Geometry: see drawing. Coordinates: mm, zero at the bounding-box minimum. A direction names the side the tool comes from. Round coordinates to 2 decimals unless told otherwise and drop trailing zeros. Loops run counter-clockwise (first coordinate to the right, second up) from the corner with the lowest first, then second, coordinate; pieces in that order, holes last. Notation, with made-up numbers: (55, -1) - (114, -1) arc R27 cw to (114, 15) - close; hole circle Ø9 at (-4.5, -26). An arc over 180 degrees is marked (long way). Write item = value, one per line. Start each with the question number.
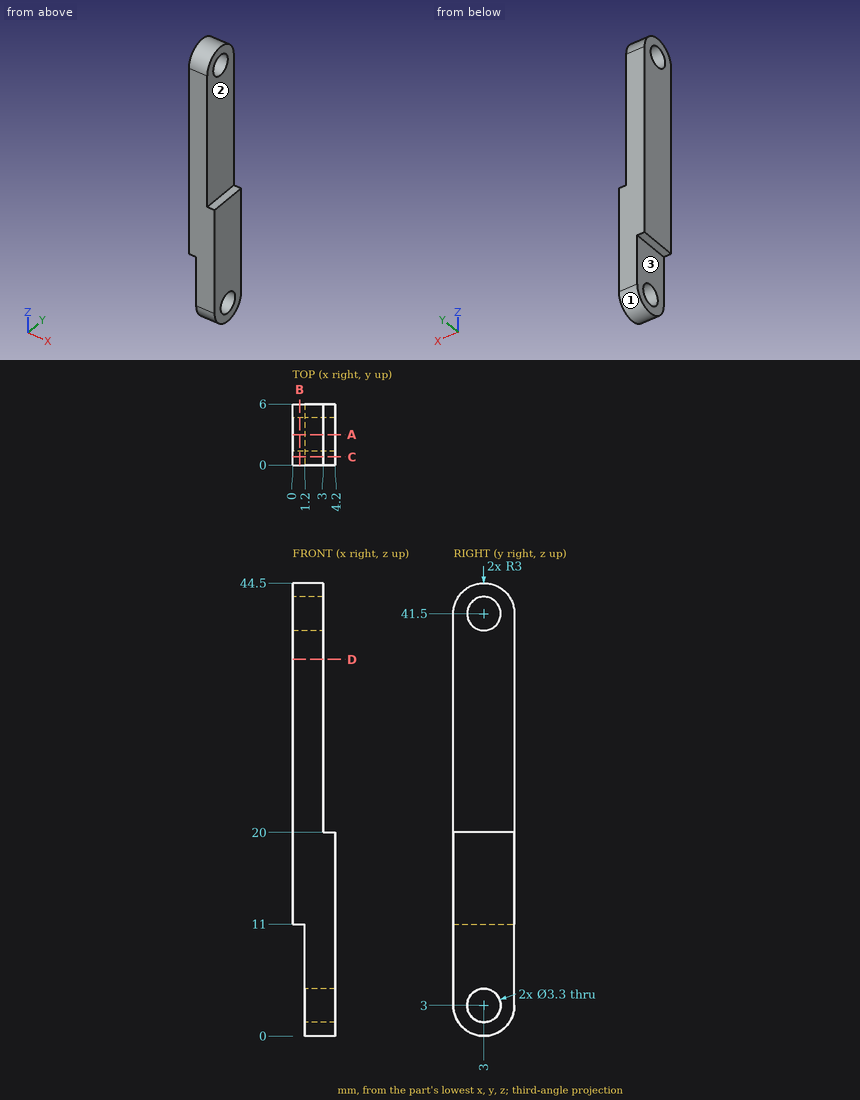
(1) Cut plane D-D (z = 37). Output: boundary loops of the cut face in (x, y), and give its area (3 significant figures).
(2) Cut plane A-A (y = 3). Output: boundary loops of the cut face in (x, z).
(3) Cut plane B-B (x = 0.7). Output: boundary loops of the cut face in (y, z), and give its area (3 significant figures).
(4) Cut plane C-C (y = 0.8). Output: boundary loops of the cut face in (x, z).
(5) Access query for the marked faces 1, 2 and 3. Directions: +Z, -Z, +X, -X, +Y, -Y. A direction counts if a zero-diameter tool reaches every point of the face in a straight line with its end or side. Return the directions, or none.
(6) Material intervals for line 1 along Y through (x, z) = (2.1, 41.5); line 2 along Z through (x, y) = (1.3, 2.1); line 3 along Z through (x, y) = (3.2, 3), sorted ascending. Write a range as from..to.
(7) Pin query (flat end, axial travel): P1, Ø3, axis at y = 3, z = 3, coming from the +X side; P2, Ø1.3, axis at x = 4, y = 3.5, coming from the +Z side; P3, Ø1.8, axis at y = 3.5, z = 4, coming from the -X side; P4, Ø1, axis at x = 0.5, y = 2.5, coming from the -Z side. Return the tip coordinate at first contact, or that it passes through.
Solution:
q1.outline = (0, 0) - (3, 0) - (3, 6) - (0, 6) - close
q1.area = 18.0 mm^2
q2.outline = (0, 11) - (1.2, 11) - (1.2, 4.65) - (4.2, 4.65) - (4.2, 20) - (3, 20) - (3, 39.85) - (0, 39.85) - close; (0, 43.15) - (3, 43.15) - (3, 44.5) - (0, 44.5) - close; (1.2, 0) - (4.2, 0) - (4.2, 1.35) - (1.2, 1.35) - close
q3.outline = (0, 11) - (6, 11) - (6, 41.5) arc R3 ccw to (0, 41.5) - close; hole circle Ø3.3 at (3, 41.5)
q3.area = 189 mm^2
q4.outline = (0, 11) - (1.2, 11) - (1.2, 0.96) - (4.2, 0.96) - (4.2, 20) - (3, 20) - (3, 43.54) - (0, 43.54) - close
q5.face_1 = -Z, +X, -X
q5.face_2 = +Z, +X, +Y, -Y
q5.face_3 = -Z, -X, +Y, -Y
q6.line_1 = 0..1.35, 4.65..6
q6.line_2 = 0.14..1.62, 4.38..40.12, 42.88..44.36
q6.line_3 = 0..1.35, 4.65..20
q7.P1 = through
q7.P2 = 20
q7.P3 = 1.2
q7.P4 = 11
